```python
from build123d import *

# Parameters (mm, degrees)
SKETCH3_R          = 1.5
CUT_EXTRUDE1_DEPTH = 14
CUT_EXTRUDE2_DEPTH = 2


with BuildPart() as part:
    # Sketch1 → Revolve1 (revolve)
    with BuildSketch(Plane.XY):
        Polygon((7, 13), (0, 13), (0, 10), (0, 0), (4, 0), (5, 1), (5, 10), (7, 10), align=None)
    revolve(axis=Axis((0, -4.570663127, 0), (0, 1, 0)))

    # Sketch3 → Cut-Extrude1 (cut, through all)
    with BuildSketch(Plane(origin=(0, 13, 0), x_dir=(1, 0, 0), z_dir=(0, 1, 0))):
        Circle(SKETCH3_R)
    extrude(amount=-CUT_EXTRUDE1_DEPTH, mode=Mode.SUBTRACT)

    # Sketch4 → Cut-Extrude2 (cut)
    with BuildSketch(Plane(origin=(0, 13, 0), x_dir=(1, 0, 0), z_dir=(0, 1, 0))):
        Polygon((2.239533559, 4.039532494), (-2.37857098, 3.959259202), (-4.618104539, -0.080273292), (-2.239533559, -4.039532494), (2.37857098, -3.959259202), (4.618104539, 0.080273292), align=None)
    extrude(amount=-CUT_EXTRUDE2_DEPTH, mode=Mode.SUBTRACT)


solid = part.part
```
Input: part model. Units: mm. Frame: model coordinates. A direction names the side the tool comes from. Coordinates: 2 decimals unless noted, no trailing zeros. Write each loop counter-clockwise with the first axis right and the second up, starting at its lowest first coordinate (ties: lowest second). Pieces come first, ordered by that corner, then holes. Notation, with made-up numbers: (-12.75, 77.25) -> (15.25, 77.25) arc R5 ccw to (15.25, 82.25) -> close; hole circle Ø3 at (32, 30.5). An arc over 180 degrees is marked (long way). Answer as a JSON object with one key per item and string values.
1. Material intervals for line 1 (Z direction, x = 0, y = 6); line 2 (Y direction, x = -1.5, z = 0.75), sorted ascending. Write a range as from..to.
Result set:
{"line 1": "z = -5..-1.5, 1.5..5", "line 2": "y = 0..11"}
2. Section B-B on x = 0. Return the cut outline in (y, z).
Result set:
{"outline": "(0, -4) -> (1, -5) -> (10, -5) -> (10, -7) -> (13, -7) -> (13, -4) -> (11, -4) -> (11, -1.5) -> (0, -1.5) -> close; (0, 1.5) -> (11, 1.5) -> (11, 4) -> (13, 4) -> (13, 7) -> (10, 7) -> (10, 5) -> (1, 5) -> (0, 4) -> close"}
3. Section D-D on z = -5.75. Return the cut outline in (x, y).
Result set:
{"outline": "(-3.99, 10) -> (3.99, 10) -> (3.99, 13) -> (-3.99, 13) -> close"}
4. Section C-C on y = 3.25. Return the cut outline in (x, z).
Result set:
{"outline": "circle Ø10 at (0, 0); hole circle Ø3 at (0, 0)"}
5. Section A-A on y = 11.75. Return the cut outline in (x, z), then the cut area to 3 significant figures.
Result set:
{"outline": "circle Ø14 at (0, 0); hole (-4.62, 0.08) -> (-2.38, -3.96) -> (2.24, -4.04) -> (4.62, -0.08) -> (2.38, 3.96) -> (-2.24, 4.04) -> close", "area": "98.5 mm2"}
6. Mould query, pull axis Z, two halves, no side actions, for faces 1 (the face through (-2, 0, 0)), 2 (the face through (-1.5, 5.58, -0.07)), 3 (the face through (6.466, 11.521, 2.681)), 4 (the face through (2, 11, 0)). Classes: released by +Z, released by -Z, zero draft, split by the parting line, or undercut.
Result set:
{"face 1": "zero draft", "face 2": "undercut", "face 3": "split by the parting line", "face 4": "undercut"}
7. First-contact query: P1, Ø6, axis at y = 6, z = -1, coming from the +X side; P2, Ø4, axis at x = 0, z = 0, coming from the +Y side. Flat tips, straight axial feed; report the tip coordinate or a pass-through.
Result set:
{"P1": "stops at x = 5", "P2": "stops at y = 11"}
8. Access query for faces 5 (the face through (-3.2, 13, 3)), 6 (the face through (2, 10, -5)), 7 (the face through (3.445, 12.014, -2.032)). Directions: +Z, -Z, +X, -X, +Y, -Y. A direction counts if a zero-diameter tool reaches every point of the face in a straight line with its end or side. Return the directions, or none.
Result set:
{"face 5": "+Z, -Z, +X, -X, +Y", "face 6": "-Y", "face 7": "+Y"}
